Can you work these out from the model? Positions are in its coordinate system, mm. A direction names the side the tool comes from. Round coordinates to 2 decimals unless told otherwise and drop trailing zeros. Write each loop counter-clockwise with the first axis right and the second up, starting at its lowest first coordinate (ties: lowest second). Pieces come first, ordered by that corner, then holes. Notation, with made-up numbers: (42, -24.75) -> (87, -24.75) arc R20 cw to (87, -20.75) -> close; hole circle Ø8 at (-3.75, -13). An arc over 180 degrees is marked (long way). Use CSV: the item, a comma, the result in double quotes.
Autodesk Inventor part; units mm, degrees
ref_plane "YZ Plane" through (0, 0, 0) normal (1, 0, 0) x (0, 1, 0)
ref_plane "XZ Plane" through (0, 0, 0) normal (0, 1, 0) x (-1, 0, 0)
ref_plane "XY Plane" through (0, 0, 0) normal (0, 0, 1) x (1, 0, 0)
sketch "Sketch1" plane through (0, 0, 0) normal (0, 1, 0) x (-1, 0, 0)
  arc A0 (77.046154, 77.046154) -> (0, 108.959716) centre (0, 0) ccw
  arc A1 (64.375202, 64.375202) -> (0, 91.040284) centre (0, 0) ccw
  line L0 (0, 113.959716) -> (0, 0)
  arc A2 (51.70425, 51.70425) -> (0, 73.120851) centre (0, 0) ccw
  arc A3 (39.033297, 39.033297) -> (0, 55.201418) centre (0, 0) ccw
  arc A4 (26.362345, 26.362345) -> (0, 37.281986) centre (0, 0) ccw
  arc A5 (70.710678, 70.710678) -> (0, 100) centre (0, 0) ccw construction
  arc A6 (13.691392, 13.691392) -> (0, 19.362553) centre (0, 0) ccw
  line L1 (0, 0) -> (80.581688, 80.581688)
  arc A7 (80.581688, 80.581688) -> (0, 113.959716) centre (0, 0) ccw
  arc A8 (10.155859, 10.155859) -> (0, 14.362553) centre (0, 0) ccw
  dimension "d8" = 45
  dimension "d0" = 17.91943
  dimension "d2" = 8.95972
  dimension "d3" = 200
  dimension "d4" = 17.91943
  dimension "d5" = 17.91943
  dimension "d6" = 17.91943
  dimension "d9" = 17.91943
  dimension "d10" = 5
  dimension "d11" = 5
extrude "Extrusion1" add sketch "Sketch1" along normal blind 5 contours L1 A1 L0 A0 | A0 L0 A7 L1 | L1 A2 L0 A1 | L1 A3 L0 A2 | L1 A4 L0 A3 | L1 A6 L0 A4 | L1 A8 L0 A6
sketch "Sketch2" plane through (-80.581688, 0, 80.581688) normal (-0.7071068, 0, -0.7071068) x (-0.7071068, 0, 0.7071068)
  line L0 (-5, 0) -> (-36.913562, 0)
  line L1 (-22.919433, 0) -> (-49.584514, 0)
  line L2 (-40.838865, 0) -> (-62.255467, 0)
  line L3 (-58.758298, 0) -> (-74.926419, 0)
  line L4 (-76.677731, 0) -> (-87.597372, 0)
  line L5 (-94.597164, 0) -> (-100.268324, 0)
  circle A0 centre (-5, 0) radius 1.65
  circle A1 centre (-22.919433, 0) radius 1.65
  circle A2 centre (-40.838865, 0) radius 1.65
  circle A3 centre (-58.758298, 0) radius 1.65
  circle A4 centre (-76.677731, 0) radius 1.65
  circle A5 centre (-94.597164, 0) radius 1.65
  point P0 (-113.959716, 0)
  dimension "d14" = 3.3
sweep "Sweep1" cut profiles "Sketch2" path "Sketch1" path curves A0 contours A0
sweep "Sweep2" cut profiles "Sketch2" path "Sketch1" path curves A1 contours A1 L0 | L0 A1
sweep "Sweep3" cut profiles "Sketch2" path "Sketch1" path curves A2 contours A2 L1 | L1 A2
sweep "Sweep4" cut profiles "Sketch2" path "Sketch1" path curves A3 contours A3 L2 | L2 A3
sweep "Sweep5" cut profiles "Sketch2" path "Sketch1" path curves A4 contours A4
sweep "Sweep6" cut profiles "Sketch2" path "Sketch1" path curves A6 contours A5
sketch "Sketch3" plane through (0, 0, 0) normal (0, -1, 0) x (1, 0, 0)
  arc A0 (0, 110.609716) -> (-78.21288, 78.21288) centre (0, 0) ccw
  line L0 (0, 113.959716) -> (0, 110.609716)
  arc A1 (0, 113.959716) -> (-80.581688, 80.581688) centre (0, 0) ccw
  line L1 (-78.21288, 78.21288) -> (-80.581688, 80.581688)
  arc A2 (0, 92.690284) -> (-65.541928, 65.541928) centre (0, 0) ccw
  line L2 (0, 107.309716) -> (0, 92.690284)
  arc A3 (0, 107.309716) -> (-75.879428, 75.879428) centre (0, 0) ccw
  line L3 (-65.541928, 65.541928) -> (-75.879428, 75.879428)
  arc A4 (0, 74.770851) -> (-52.870976, 52.870976) centre (0, 0) ccw
  line L4 (0, 89.390284) -> (0, 74.770851)
  arc A5 (0, 89.390284) -> (-63.208476, 63.208476) centre (0, 0) ccw
  line L5 (-52.870976, 52.870976) -> (-63.208476, 63.208476)
  arc A6 (0, 56.851418) -> (-40.200023, 40.200023) centre (0, 0) ccw
  line L6 (0, 71.470851) -> (0, 56.851418)
  arc A7 (0, 71.470851) -> (-50.537523, 50.537523) centre (0, 0) ccw
  line L7 (-40.200023, 40.200023) -> (-50.537523, 50.537523)
  arc A8 (0, 38.931986) -> (-27.529071, 27.529071) centre (0, 0) ccw
  line L8 (0, 53.551418) -> (0, 38.931986)
  arc A9 (0, 53.551418) -> (-37.866571, 37.866571) centre (0, 0) ccw
  line L9 (-27.529071, 27.529071) -> (-37.866571, 37.866571)
  arc A10 (0, 21.012553) -> (-14.858119, 14.858119) centre (0, 0) ccw
  line L10 (0, 35.631986) -> (0, 21.012553)
  arc A11 (0, 35.631986) -> (-25.195619, 25.195619) centre (0, 0) ccw
  line L11 (-14.858119, 14.858119) -> (-25.195619, 25.195619)
  arc A12 (0, 17.712553) -> (-12.524666, 12.524666) centre (0, 0) ccw
  line L12 (-10.155859, 10.155859) -> (-12.524666, 12.524666)
  arc A13 (0, 14.362553) -> (-10.155859, 10.155859) centre (0, 0) ccw
  line L13 (0, 17.712553) -> (0, 14.362553)
extrude "Extrusion2" add sketch "Sketch3" along normal blind 1.65
equation "\"d0\" = d25"
equation "\"d2\" = 0.5 * d25"
equation "\"d4\" = d25"
equation "\"d5\" = d4"
equation "\"d6\" = d5"
equation "\"d9\" = d6"
equation "\"d14\" = trackDiameter"
equation "\"d28\" = 0.5 * trackDiameter"
properties part number "Curved Track Builder"
Q1. If we mould it in two halves opening along Z, with no side actions, what happens to faces 1 (the face through (-28.99, -0.81, 68.92)), 2 (the face through (-31, 5, 74)), 3 (the face through (-45, 2, 45))? For each: released by +Z, released by -Z, zero draft, split by the parting line, or undercut.
Resolved:
face 1,"undercut"
face 2,"zero draft"
face 3,"released by -Z"
Q2. Suppose I cut it at A-A (y = 3.5). Write out the boundary of the cut face in (x, z), and give its area (3 significant figures).
Resolved:
outline,"(-80.58, 80.58) -> (-10.16, 10.16) arc R14.36 cw to (0, 14.36) -> (0, 113.96) arc R113.96 ccw to start"
area,"5,020 mm^2"
Q3. Will these pins go through, and if not, where does the flat tip stop? P1, Ø3, axis at x = -13.5, y = -0.5, coming from the +Z side; P2, Ø2, axis at y = 3, z = 24, coming from the -X side.
Resolved:
P1,"stops at z = 113.33"
P2,"stops at x = -25"
Q4. Please list where these lines run through material, in increasing order: probe 1 along Z at (x, y) = (-48, 1); probe 2 along Z at (x, y) = (-67, -0.5); probe 3 along Y at (x, z) = (-49, 97).
Resolved:
probe 1,"z = 48 to 53.41, 56.89 to 75.81, 78.9 to 96.35, 99.28 to 103.36"
probe 2,"z = 67 to 83.82, 88.01 to 92.18"
probe 3,"y = 1.63 to 5"
Q5. On a 3-axis mill with a long thin cutter (end or side, diameter ignored), from which of +Z, -Z, +X, -X, +Y, -Y can I reach the whole of each face in a straight line? I mean faces 4 (the face through (-41.61, -0.813, 98.914)), 5 (the face through (-10, -1.65, 25)). Say none if no direction works.
Resolved:
face 4,"-Y"
face 5,"+Z, -Z, +X, -X, -Y"
